Geometry: see drawing. Coordinates: mm, zero at the bounding-box minimum. A direction names the side the tool comes from. Coordinates: 2 decimals unless noted, no trailing zeros. Loops run counter-clockwise (first coordinate to the right, second up) from the corner with the lowest first, then second, coordinate; pieces in that order, holes last. Notation, with made-up numbers: (17.5, 11) -> (66.5, 11) arc R9 cw to (66.5, 28) -> close; hole circle Ø3 at (72, 51.25). An arc over 180 degrees is marked (long way). One line per item, written item: value. Start each with the question number.
Item 1: Section query D-D on x = 3.8. Return loops of the section in (y, z) (3 decimals).
Item 2: Contact query for flat-ended pins moving along their axis: pin 1 Ø0.8 at (x, z) = (3, 4.5) entering from +Y; pin 2 Ø1.3 at (x, y) = (4.5, 2.5) entering from -Z. Output: stop coordinate, or through.
Item 3: Section query C-C on z = 4. Return loops of the section in (x, y).
Item 4: Section query B-B on y = 1.5. Return loops of the section in (x, z) (3 decimals).
Item 5: Ray query, probe 1 along X at (y, z) = (4.25, 2); probe 2 along Y at (x, z) = (3, 5.5); probe 3 along Z at (x, y) = (2.2, 2.5) (3 decimals). Return the intervals inside material, ascending. Write a range as from..to.
Item 6: Set-up query: the marked faces 5, 6, 7 and 8. Return all of +Z, -Z, +X, -X, +Y, -Y with unobstructed straight access to the full face (end or side cutting, diameter ignored); none if empty.
Item 7: Section query A-A on z = 1.75. Return loops of the section in (x, y).
Item 8: Mould query, pull axis X, two halves, no side actions, for the marked faces 1, 2, 3 and 4. Classes: +X half, -X half, draft (parallel to the pull), parting line (faces both ways), or undercut.
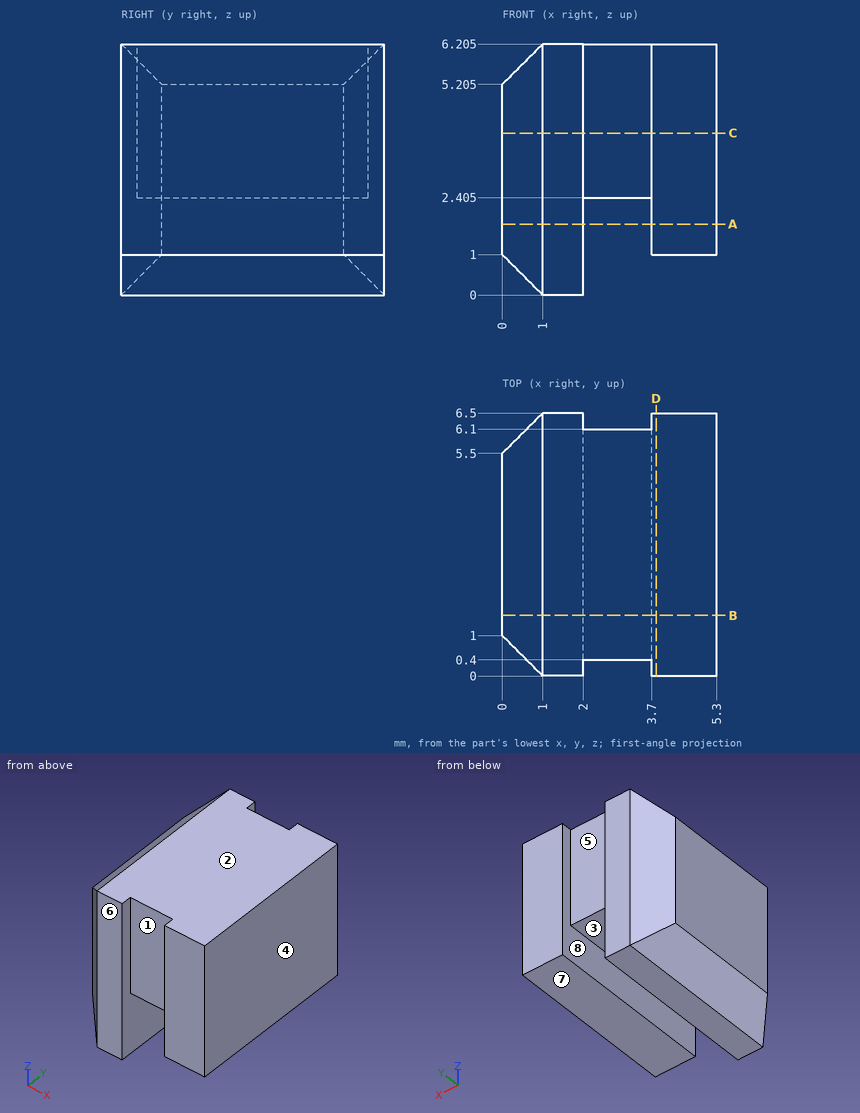
Reply:
1. outline: (0, 1) -> (6.5, 1) -> (6.5, 6.205) -> (0, 6.205) -> close
2. pin 1: stops at y = 6.1
2. pin 2: stops at z = 1
3. outline: (0, 1) -> (1, 0) -> (2, 0) -> (2, 0.4) -> (3.7, 0.4) -> (3.7, 0) -> (5.3, 0) -> (5.3, 6.5) -> (3.7, 6.5) -> (3.7, 6.1) -> (2, 6.1) -> (2, 6.5) -> (1, 6.5) -> (0, 5.5) -> close
4. outline: (0, 1) -> (1, 0) -> (2, 0) -> (2, 2.405) -> (3.7, 2.405) -> (3.7, 1) -> (5.3, 1) -> (5.3, 6.205) -> (1, 6.205) -> (0, 5.205) -> close
5. probe 1: x = 0..2, 3.7..5.3
5. probe 2: y = 0.4..6.1
5. probe 3: z = 2.405..6.205
6. face 5: +Z, -Z, +Y
6. face 6: +Z, -Z, +X, -X, -Y
6. face 7: -Z, +X, +Y, -Y
6. face 8: -Z
7. outline: (0, 1) -> (1, 0) -> (2, 0) -> (2, 6.5) -> (1, 6.5) -> (0, 5.5) -> close; (3.7, 0) -> (5.3, 0) -> (5.3, 6.5) -> (3.7, 6.5) -> close
8. face 1: undercut
8. face 2: draft
8. face 3: undercut
8. face 4: +X half
